Answer from the drawing. Dimensions are ordinates in mm from the lowest x, y and z of the part. A direction names the side the tool comes from. Round coordinates to 2 decimals unless told otherwise and drop trailing zeros. Loops run counter-clockwise (first coordinate to the right, second up) from the corner with the lowest first, then second, coordinate; pieces in that order, holes last. Notation, with made-up numbers: M -3.75,-13.75 L 42.25,-13.75 A14 ccw 42.25,-5.75 Z; hole C -28,38.5 d1. An arc over 180 degrees is marked long. Answer as CSV lines item,"result".
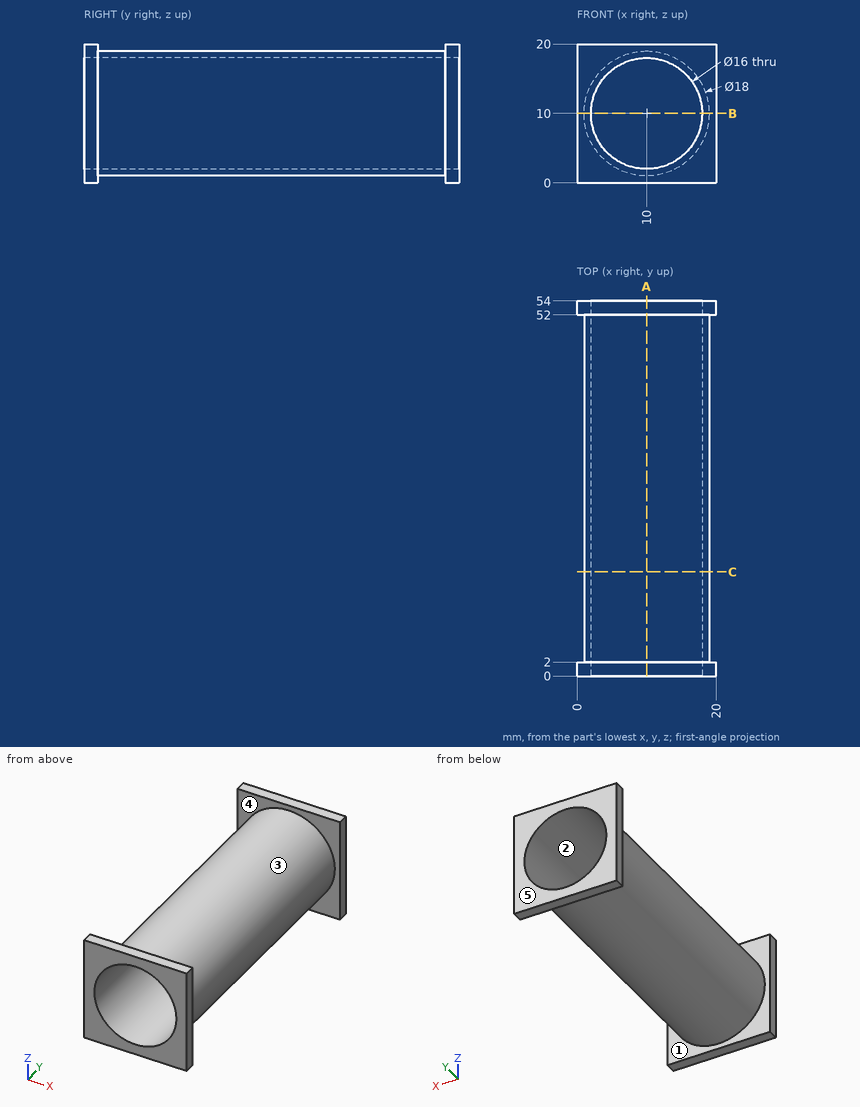
1) Determine the mould class of the marked faces 1, 2 and 3 for opening direction X: released by +X, released by -X, zero draft, split by the parting line, or undercut.
Evaluation:
face 1,"zero draft"
face 2,"undercut"
face 3,"split by the parting line"
2) Each of these flat-tipped pins is pushed along its axis until it touches: P1, Ø5, axis at y = 21, z = 12.5, coming from the +X side; P2, Ø1, axis at x = 18, y = 39.5, coming from the +Z side; P3, Ø3, axis at x = 6, y = 35, coming from the +Z side; P4, Ø10, axis at x = 16.5, z = 12, coming from the +Y side. Where does it stop, or does it pass through?
Evaluation:
P1,"stops at x = 19"
P2,"stops at z = 14.97"
P3,"stops at z = 18.65"
P4,"stops at y = 54"
3) Find section C-C, the plane y = 15. Give the vertices of the cut face in (x, z), then the cut area to 3 significant figures.
Evaluation:
outline,"C 10,10 d18; hole C 10,10 d16"
area,"53.4 mm^2"
4) Find section A-A, the plane x = 10. Give the vertices of the cut face in (y, z).
Evaluation:
outline,"M 0,0 L 2,0 L 2,1 L 52,1 L 52,0 L 54,0 L 54,2 L 0,2 Z; M 0,18 L 54,18 L 54,20 L 52,20 L 52,19 L 2,19 L 2,20 L 0,20 Z"
5) Find section B-B, the plane z = 10. Give the vertices of the cut face in (x, y), then the cut area to 3 significant figures.
Evaluation:
outline,"M 0,0 L 2,0 L 2,54 L 0,54 L 0,52 L 1,52 L 1,2 L 0,2 Z; M 18,0 L 20,0 L 20,2 L 19,2 L 19,52 L 20,52 L 20,54 L 18,54 Z"
area,"116 mm^2"
6) Straight lines are drawn through the part: line 1 (Y direction, x = 19.25, z = 19.25); line 2 (Z direction, x = 9.75, y = 46). For each, find the intervals that lie inside material, in ascending order.
Evaluation:
line 1,"y = 0 to 2, 52 to 54"
line 2,"z = 1 to 2, 18 to 19"
7) A tool of negligible diameter and unlimited length cuts with its end or side. For the marked faces 4 and 5, from which of +Z, -Z, +X, -X, +Y, -Y can it reach the whole face along a straight path? Write none if from no direction.
Evaluation:
face 4,"none"
face 5,"+Z, -Z, +X, -X, +Y"
